Source: CAD feature listing. Evaluate the final solid. Frame: model axes, mm. A direction names the side the tool comes from. Give positions to 0.01 mm unless a question says otherwise; leave off trailing zeros. Order: outer loops, then holes, each group sorted by start corner. A loop starts at its lowest first (then second) coordinate and runs counter-clockwise, first axis right, second up. Notation, with made-up numbers: (59.25, 39.5) - (105.25, 39.5) arc R13 ccw to (105.25, 43.5) - close; hole circle Ø7 at (56.25, 27). An arc over 180 degrees is marked (long way). One line per item, written item: value. Start each with the question number.
from build123d import *

# Parameters (mm, degrees)
SKETCH1_W           = 35
SKETCH1_H           = 12
BOSS_EXTRUDE1_DEPTH = 20
SKETCH2_W           = 35
SKETCH2_H           = 12
BOSS_EXTRUDE2_DEPTH = 10
CUT_EXTRUDE1_DEPTH  = 12
FILLET1_R           = 12
SKETCH5_R           = 15
SKETCH5_R_2         = 12
BOSS_EXTRUDE3_DEPTH = 10
SKETCH6_W           = 35
SKETCH6_H           = 15
BOSS_EXTRUDE4_DEPTH = 2
SKETCH7_W           = 35
SKETCH7_H           = 12
BOSS_EXTRUDE5_DEPTH = 10
SKETCH8_W           = 35
SKETCH8_H           = 40
BOSS_EXTRUDE6_DEPTH = 10
SKETCH10_R          = 11.2
CUT_EXTRUDE2_DEPTH  = 7
SKETCH11_R          = 8
CUT_EXTRUDE3_DEPTH  = 3
BOSS_EXTRUDE7_DEPTH = 12
BOSS_EXTRUDE8_DEPTH = 12
SKETCH14_W          = 12
SKETCH14_H          = 5
BOSS_EXTRUDE9_DEPTH = 5


with BuildPart() as part:
    # Sketch1 → Boss-Extrude1 (new body)
    with BuildSketch(Plane(origin=(0, 0, 0), x_dir=(1, 0, 0), z_dir=(0, 1, 0))):
        Rectangle(SKETCH1_W, SKETCH1_H)
    extrude(amount=BOSS_EXTRUDE1_DEPTH)

    # Sketch2 → Boss-Extrude2 (add)
    with BuildSketch(Plane(origin=(0, 20, 0), x_dir=(1, 0, 0), z_dir=(0, 1, 0))):
        Rectangle(SKETCH2_W, SKETCH2_H)
    extrude(amount=BOSS_EXTRUDE2_DEPTH)

    # Sketch4 → Cut-Extrude1 (cut)
    with BuildSketch(Plane(origin=(0, 0, -6), x_dir=(-1, 0, 0), z_dir=(0, 0, -1))):
        with BuildLine():
            ThreePointArc((8, 15), (0, 23), (-8, 15))
            Line((-8, 15), (8, 15))
        make_face()
        with BuildLine():
            Line((8, 15), (-8, 15))
            ThreePointArc((-8, 15), (0, 7), (8, 15))
        make_face()
    extrude(amount=-CUT_EXTRUDE1_DEPTH, mode=Mode.SUBTRACT)

    # Fillet1
    fillet1_edges = [part.edges().sort_by_distance(p)[0] for p in [
        (-17.5, 30, 0),
        (17.5, 30, 0),
    ]]
    fillet(fillet1_edges, radius=FILLET1_R)

    # Sketch5 → Boss-Extrude3 (add)
    with BuildSketch(Plane(origin=(0, 0, -6), x_dir=(-1, 0, 0), z_dir=(0, 0, -1))):
        with Locations(Location((0, 15, 0), (0, 0, 270))):
            Circle(SKETCH5_R)
        with Locations((0, 15)):
            Circle(SKETCH5_R_2, mode=Mode.SUBTRACT)
    extrude(amount=BOSS_EXTRUDE3_DEPTH)

    # Sketch6 → Boss-Extrude4 (add)
    with BuildSketch(Plane.XZ):
        with Locations((0, 1.5)):
            Rectangle(SKETCH6_W, SKETCH6_H)
    extrude(amount=BOSS_EXTRUDE4_DEPTH)

    # Sketch7 → Boss-Extrude5 (add)
    with BuildSketch(Plane.XZ.offset(2)):
        Rectangle(SKETCH7_W, SKETCH7_H)
    extrude(amount=BOSS_EXTRUDE5_DEPTH)

    # Sketch8 → Boss-Extrude6 (add)
    with BuildSketch(Plane.XZ.offset(12)):
        with Locations((0, 14)):
            Rectangle(SKETCH8_W, SKETCH8_H)
    extrude(amount=BOSS_EXTRUDE6_DEPTH)

    # Sketch10 → Cut-Extrude2 (cut)
    with BuildSketch(Plane.XZ.offset(22)):
        with Locations(Location((0, 14, 0), (0, 0, 270))):
            Circle(SKETCH10_R)
    extrude(amount=-CUT_EXTRUDE2_DEPTH, mode=Mode.SUBTRACT)

    # Sketch11 → Cut-Extrude3 (cut)
    with BuildSketch(Plane.XZ.offset(15)):
        with Locations(Location((0, 14, 0), (0, 0, 270))):
            Circle(SKETCH11_R)
    extrude(amount=-CUT_EXTRUDE3_DEPTH, mode=Mode.SUBTRACT)

    # Sketch12 → Boss-Extrude7 (add)
    with BuildSketch(Plane(origin=(0, 0, -6), x_dir=(-1, 0, 0), z_dir=(0, 0, -1))):
        Polygon((17.5, -22), (17.5, -7), (25.915107819, -1.597596795), (25.915107819, -16.597596795), align=None)
    extrude(amount=-BOSS_EXTRUDE7_DEPTH)

    # Sketch13 → Boss-Extrude8 (add)
    with BuildSketch(Plane.XY.offset(6)):
        Polygon((-17.5, -22), (-17.5, -7), (-59.575539097, 20.012016024), (-59.575539097, 5.012016024), align=None)
    extrude(amount=BOSS_EXTRUDE8_DEPTH)

    # Sketch14 → Boss-Extrude9 (add)
    with BuildSketch(Plane(origin=(-17.5, 0, 0), x_dir=(0, 0, -1), z_dir=(1, 0, 0))):
        with Locations((-12, -9.5)):
            Rectangle(SKETCH14_W, SKETCH14_H)
    extrude(amount=BOSS_EXTRUDE9_DEPTH)


solid = part.part
1. Section B-B on y = 15. Return the cut outline in (x, z).
2. Ray query, L1, parallel to Y at x = 0, z = 1.75; L2, parallel to Z at x = 10.5, y = 17; L3, parallel to Z at x = -28.5, y = -2. Return the intervals inside material, ascending.
3. Draft query along X for faces 6 (the cylindrical face through (-4.868, -13.521, 20.349)), 7 (the cylindrical face through (11.99, 15.53, -10.93)), 8 (the flat face through (-59.576, 13, 12)), 9 (the flat face through (0, -2, 8)). Return one class per face: pulls with the +X half, pulls with the -X half, needs draft (parallel to the pull), parting line crosses it, or undercut.
4. Section A-A on z = 0.5. Return the cut outline in (x, y).
5. Contact query for flat-ended pins moving along their axis: pin 1 Ø18.5 at (x, z) = (0, 14) entering from +Y; pin 2 Ø1 at (x, z) = (-9.5, 11.5) entering from +Y; pin 3 Ø14.5 at (x, y) = (0, 15) entering from -Z; pin 4 Ø24 at (x, y) = (1, 16) entering from +Z. Output: stop coordinate, or through.
6. Section D-D on z = 14. Return the cut outline in (x, y).
7. Section C-C on x = 2. Count the separate pieces of the cut face and the enclosed holes in it, then the cut area to 3 significant figures.
8. Set-up query: faces 1 (the flat face through (8, 17, -6)), 2 (the flat face through (0, 0, 8)), 3 (the flat face through (-12.5, -9, 12)), 4 (the flat face through (0, -17, 34)), 5 (the flat face through (-43, 2, 6)). Return all of +Z, -Z, +X, -X, +Y, -Y with unobstructed straight access to the full face (end or side cutting, diameter ignored); none if empty.
Data:
1. outline: (-59.58, 6) - (-51.77, 6) - (-51.77, 18) - (-59.58, 18) - close; (-17.5, -6) - (-15, -6) - (-15, -16) - (-12, -16) - (-12, -6) - (-8, -6) - (-8, 6) - (-17.5, 6) - close; (8, -6) - (12, -6) - (12, -16) - (15, -16) - (15, -6) - (17.5, -6) - (17.5, 6) - (8, 6) - close
2. L1: y = -22 to 7, 23 to 30
2. L2: z = -6 to 6
2. L3: z = 6 to 18
3. face 6: undercut
3. face 7: undercut
3. face 8: pulls with the -X half
3. face 9: needs draft
4. outline: (-25.92, -16.6) - (-17.5, -22) - (17.5, -22) - (17.5, 18) arc R12 ccw to (5.5, 30) - (-5.5, 30) arc R12 ccw to (-17.5, 18) - (-17.5, -7) - (-25.92, -1.6) - close; hole circle Ø16 at (0, 15)
5. pin 1: stops at y = 30
5. pin 2: stops at y = -12
5. pin 3: passes through
5. pin 4: stops at z = 6
6. outline: (-59.58, 5.01) - (-17.5, -22) - (-11.2, -22) - (-11.2, -15) - (-8, -15) - (-8, -12) - (-12.5, -12) - (-12.5, -7) - (-17.5, -7) - (-59.58, 20.01) - close; (8, -15) - (11.2, -15) - (11.2, -22) - (17.5, -22) - (17.5, -12) - (8, -12) - close
7. separate pieces: 3
7. enclosed holes: 0
7. area: 584 mm2
8. face 1: -Z
8. face 2: +Z, +X, +Y
8. face 3: +Z, +X
8. face 4: +Z, +X, -X, +Y, -Y
8. face 5: -Z, -X, +Y, -Y
